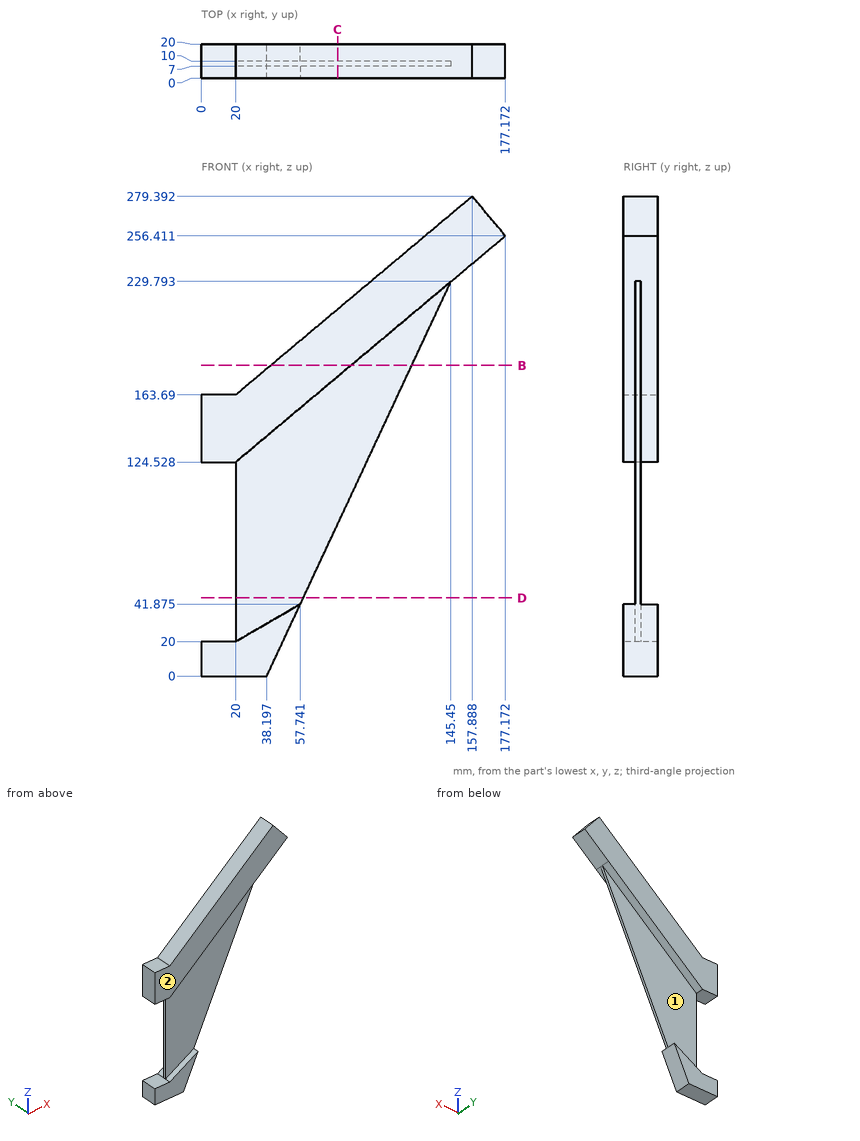
Here's the drawing with two shaded views (mm, measured from the low corner). I have some questions. Give positions to 0.01 mm unless a question says otherwise; leave off trailing zeros. Write each loop counter-clockwise with the first axis right and the second up, starting at its lowest first coordinate (ties: lowest second). Pieces come first, ordered by that corner, then holes. Notation, with made-up numbers: (-7.5, 41) -> (27.5, 41) arc R25 ccw to (27.5, 56) -> close; hole circle Ø8 at (-6, 50.25). An arc over 180 degrees is marked (long way). Answer as a JSON object with one key per item and string values. Group by question number.
Item 1: Suppose I cut it at C-C (x = 79.5). Please give me the cut outline in (y, z) (1 decimal).
Item 2: I'm going to push flat-ended pins straight in: P1, Ø10, axis at x = 11.5, y = 11.5, coming from the +Z side; P2, Ø0.9, axis at y = 8.5, z = 82, coming from the -X side; P3, Ø6, axis at x = 6.5, y = 14, coming from the -Z side; P4, Ø5, axis at x = 32.5, y = 14.5, coming from the +Z side. Where does each tip first touch, or does it pass through?
Item 3: Suppose I cut it at B-B (z = 181). Please give me the cut outline in (x, y), plus the area to 3 significant figures.
Item 4: We'd pull the mould along Z, two halves only. Please class the marked faces 1 and 2: +Z half, -Z half, draft (parallel to the pull), parting line (faces both ways), or undercut.
Item 5: Suppose I cut it at D-D (z = 45.5). Please give me the cut outline in (x, y), plus the area to 3 significant figures.
Item 6: Please list where these lines run through material, in increasing order: line 1 (Z direction, x = 14.5, y = 16.5); line 2 (Y direction, x = 64.5, z = 71); line 3 (Z direction, x = 53, y = 14.5) (1 decimal). Write a range as [from, to].
Findings:
{
 "1": {"outline": "(0, 174.5) -> (7, 174.5) -> (7, 88.5) -> (10, 88.5) -> (10, 174.5) -> (20, 174.5) -> (20, 213.6) -> (0, 213.6) -> close"},
 "2": {"P1": "stops at z = 163.69", "P2": "stops at x = 20", "P3": "stops at z = 0", "P4": "stops at z = 176.28"},
 "3": {"outline": "(40.63, 0) -> (87.3, 0) -> (87.3, 7) -> (122.68, 7) -> (122.68, 10) -> (87.3, 10) -> (87.3, 20) -> (40.63, 20) -> close", "area": "1,040 mm²"},
 "4": {"face 1": "undercut", "face 2": "draft"},
 "5": {"outline": "(20, 7) -> (59.43, 7) -> (59.43, 10) -> (20, 10) -> close", "area": "118 mm²"},
 "6": {"line 1": "z = [0, 20], [124.53, 163.69]", "line 2": "y = [7, 10]", "line 3": "z = [31.7, 39.1], [152.2, 191.4]"}
}
